from build123d import *

# Parameters (mm, degrees)
SKETCH1_W           = 6.096
SKETCH1_H           = 5.334
SKETCH1_R           = 2.122
BOSS_EXTRUDE1_DEPTH = 30.48
FILLET1_R           = 0.508


with BuildPart() as part:
    # Sketch1 → Boss-Extrude1 (new body)
    with BuildSketch(Plane(origin=(0, 0, 0), x_dir=(1, 0, 0), z_dir=(0, 1, 0))):
        Rectangle(SKETCH1_W, SKETCH1_H)
        with Locations(Location((0, 0, 0), (0, 0, 90))):
            Circle(SKETCH1_R, mode=Mode.SUBTRACT)
    extrude(amount=BOSS_EXTRUDE1_DEPTH)

    # Fillet1
    fillet1_edges = [part.edges().sort_by_distance(p)[0] for p in [
        (3.048, 15.24, 2.667),
        (-3.048, 15.24, 2.667),
        (-3.048, 15.24, -2.667),
        (3.048, 15.24, -2.667),
    ]]
    fillet(fillet1_edges, radius=FILLET1_R)


solid = part.part
Could you check a few things on this model? Use its own coordinates, in mm. Give positions to 0.01 mm unless a question says otherwise; leave off trailing zeros. Order: outer loops, then holes, each group sorted by start corner. A loop starts at its lowest first (then second) coordinate and runs counter-clockwise, first axis right, second up.
1. Suppose I cut it at C-C (y = 13). Write out the boundary of the cut face in (x, z).
Answers below:
outline: (-3.05, -2.16) arc R0.51 ccw to (-2.54, -2.67) - (2.54, -2.67) arc R0.51 ccw to (3.05, -2.16) - (3.05, 2.16) arc R0.51 ccw to (2.54, 2.67) - (-2.54, 2.67) arc R0.51 ccw to (-3.05, 2.16) - close; hole circle Ø4.24 at (0, 0)
2. Thinking about a two-plate mould opening in Z: for faces 1 (the flat face through (-1.4, 30.48, -1.8)), 2 (the cylindrical face through (-0.637, 15.027, -2.024)), 3 (the flat face through (0, 15, -2.667)), which applies, +Z half, -Z half, draft (parallel to the pull), parting line (faces both ways), or undercut?
Answers below:
face 1: draft
face 2: undercut
face 3: -Z half
3. For pin 1 (1 mm diameter, centred on x = 2, z = 1, fed in from -Y), with a flat end and sliding along its axis, tell me the tip position at first contact or that it passes through.
Answers below:
pin 1: stops at y = 0
4. Suppose I cut it at B-B (x = 0). Write out the boundary of the cut face in (y, z), plus the area to 3 significant figures.
Answers below:
outline: (0, -2.67) - (30.48, -2.67) - (30.48, -2.12) - (0, -2.12) - close; (0, 2.12) - (30.48, 2.12) - (30.48, 2.67) - (0, 2.67) - close
area: 33.2 mm2
5. I need wall thicknesses on L1, parallel to X at y = 13.5, z = 0; L2, parallel to Z at x = 0.5, y = 27; L3, parallel to Z at x = -1.25, y = 4. Which ranges of each line are inside material? Lowest first, please.
Answers below:
L1: x = -3.05 to -2.12, 2.12 to 3.05
L2: z = -2.67 to -2.06, 2.06 to 2.67
L3: z = -2.67 to -1.71, 1.71 to 2.67
6. Suppose I cut it at A-A (z = 0). Write out the boundary of the cut face in (x, y).
Answers below:
outline: (-3.05, 0) - (-2.12, 0) - (-2.12, 30.48) - (-3.05, 30.48) - close; (2.12, 0) - (3.05, 0) - (3.05, 30.48) - (2.12, 30.48) - close
